```python
from build123d import *

# Parameters (mm, degrees)
BOSS_EXTRUDE1_DEPTH                     = 40
CUT_EXTRUDE3_REACH                      = 349.563
SKETCH2_W                               = 10
SKETCH2_H                               = 8
FILLET1_RADIUS                          = 15
FILLET1_LENGTH                          = 15
SKETCH3_R                               = 5
CUT_EXTRUDE4_DEPTH                      = 15
CUT_EXTRUDE5_REACH                      = 349.394
CBORE_FOR_M5_HEX_HEAD_BOLT1_D           = 10
CBORE_FOR_M5_HEX_HEAD_BOLT1_CBORE_D     = 15
CBORE_FOR_M5_HEX_HEAD_BOLT1_CBORE_DEPTH = 8
CUT_EXTRUDE6_DEPTH                      = 40


with BuildPart() as part:
    # Sketch1 → Boss-Extrude1 (new, symmetric)
    with BuildSketch(Plane.YZ):
        with BuildLine():
            Line((0, 0), (47.251760651, 0))
            ThreePointArc((47.251760651, 0), (58.870710689, 4.252272915), (65, 15))
            Line((65, 15), (196.846599289, 15))
            ThreePointArc((196.846599289, 15), (222.463976204, 19.510639101), (245, 32.5))
            Line((245, 32.5), (280, 32.5))
            Line((280, 32.5), (300, 12.5))
            Line((300, 12.5), (300, -12.5))
            Line((300, -12.5), (340, -12.5))
            Line((340, -12.5), (340, -27.5))
            Line((340, -27.5), (245, -27.5))
            add(Edge.make_bspline(
                [(179, -15), (212.333333333, -15), (211.666666667, -27.5), (245, -27.5)],
                knots=[0, 0, 0, 0, 1, 1, 1, 1], degree=3))
            Line((179, -15), (0, -15))
            Line((0, -15), (0, 0))
        make_face()
    extrude(amount=BOSS_EXTRUDE1_DEPTH, both=True)

    # Cut-Extrude3: up to this face of the body (flat: up to its plane)
    cut_extrude3_end = Plane(part.part.faces().sort_by_distance((0, 292.5, -27.5))[0])
    # Sketch2 → Cut-Extrude3 (cut, up to the picked face)
    with BuildSketch(Plane.XY.offset(32.5), mode=Mode.PRIVATE) as cut_extrude3_sk1:
        with BuildLine():
            Line((15, 202.853988128), (15, 0))
            Line((15, 0), (40, 0))
            Line((40, 0), (40, 47.251760651))
            Line((40, 47.251760651), (40, 245))
            Line((40, 245), (22.765371804, 245))
            Line((22.765371804, 245), (18.407417371, 228.735892638))
            ThreePointArc((18.407417371, 228.735892638), (15.855513863, 215.90660735), (15, 202.853988128))
        make_face()
    cut_extrude3_tool1 = split(extrude(cut_extrude3_sk1.sketch, amount=-CUT_EXTRUDE3_REACH, mode=Mode.PRIVATE), bisect_by=cut_extrude3_end, keep=Keep.BOTH, mode=Mode.PRIVATE)
    # Sketch2 → Cut-Extrude3 (cut, up to the picked face)
    with BuildSketch(Plane.XY.offset(32.5), mode=Mode.PRIVATE) as cut_extrude3_sk2:
        with BuildLine():
            Line((-40, 0), (-15, 0))
            Line((-15, 0), (-15, 202.853988128))
            ThreePointArc((-15, 202.853988128), (-15.855513863, 215.90660735), (-18.407417371, 228.735892638))
            Line((-18.407417371, 228.735892638), (-22.765371804, 245))
            Line((-22.765371804, 245), (-40, 245))
            Line((-40, 245), (-40, 0))
        make_face()
    cut_extrude3_tool2 = split(extrude(cut_extrude3_sk2.sketch, amount=-CUT_EXTRUDE3_REACH, mode=Mode.PRIVATE), bisect_by=cut_extrude3_end, keep=Keep.BOTH, mode=Mode.PRIVATE)
    # Sketch2 → Cut-Extrude3 (cut, up to the picked face)
    with BuildSketch(Plane.XY.offset(32.5), mode=Mode.PRIVATE) as cut_extrude3_sk3:
        Polygon((30, 272), (22.765371804, 245), (40, 245), (40, 272), align=None)
    cut_extrude3_tool3 = split(extrude(cut_extrude3_sk3.sketch, amount=-CUT_EXTRUDE3_REACH, mode=Mode.PRIVATE), bisect_by=cut_extrude3_end, keep=Keep.BOTH, mode=Mode.PRIVATE)
    # Sketch2 → Cut-Extrude3 (cut, up to the picked face)
    with BuildSketch(Plane.XY.offset(32.5), mode=Mode.PRIVATE) as cut_extrude3_sk4:
        Polygon((-40, 272), (-40, 245), (-22.765371804, 245), (-30, 272), align=None)
    cut_extrude3_tool4 = split(extrude(cut_extrude3_sk4.sketch, amount=-CUT_EXTRUDE3_REACH, mode=Mode.PRIVATE), bisect_by=cut_extrude3_end, keep=Keep.BOTH, mode=Mode.PRIVATE)
    # Sketch2 → Cut-Extrude3 (cut, up to the picked face)
    with BuildSketch(Plane.XY.offset(32.5), mode=Mode.PRIVATE) as cut_extrude3_sk5:
        with BuildLine():
            Line((30, 300), (30, 280))
            Line((30, 280), (40, 280))
            Line((40, 280), (40, 340))
            Line((40, 340), (18.5, 340))
            ThreePointArc((18.5, 340), (35.838126061, 329.969422485), (35.78511038, 309.938938469))
            Line((35.78511038, 309.938938469), (35.773706219, 309.919345885))
            Line((35.773706219, 309.919345885), (30, 300))
        make_face()
    cut_extrude3_tool5 = split(extrude(cut_extrude3_sk5.sketch, amount=-CUT_EXTRUDE3_REACH, mode=Mode.PRIVATE), bisect_by=cut_extrude3_end, keep=Keep.BOTH, mode=Mode.PRIVATE)
    # Sketch2 → Cut-Extrude3 (cut, up to the picked face)
    with BuildSketch(Plane.XY.offset(32.5), mode=Mode.PRIVATE) as cut_extrude3_sk6:
        with Locations((35, 276)):
            Rectangle(SKETCH2_W, SKETCH2_H)
    cut_extrude3_tool6 = split(extrude(cut_extrude3_sk6.sketch, amount=-CUT_EXTRUDE3_REACH, mode=Mode.PRIVATE), bisect_by=cut_extrude3_end, keep=Keep.BOTH, mode=Mode.PRIVATE)
    # Sketch2 → Cut-Extrude3 (cut, up to the picked face)
    with BuildSketch(Plane.XY.offset(32.5), mode=Mode.PRIVATE) as cut_extrude3_sk7:
        with Locations((-35, 276)):
            Rectangle(SKETCH2_W, SKETCH2_H)
    cut_extrude3_tool7 = split(extrude(cut_extrude3_sk7.sketch, amount=-CUT_EXTRUDE3_REACH, mode=Mode.PRIVATE), bisect_by=cut_extrude3_end, keep=Keep.BOTH, mode=Mode.PRIVATE)
    # Sketch2 → Cut-Extrude3 (cut, up to the picked face)
    with BuildSketch(Plane.XY.offset(32.5), mode=Mode.PRIVATE) as cut_extrude3_sk8:
        with BuildLine():
            Line((-40, 340), (-40, 280))
            Line((-40, 280), (-30, 280))
            Line((-30, 280), (-30, 300))
            Line((-30, 300), (-35.773706219, 309.919345885))
            Line((-35.773706219, 309.919345885), (-35.78511038, 309.938938469))
            ThreePointArc((-35.78511038, 309.938938469), (-35.838126061, 329.969422485), (-18.5, 340))
            Line((-18.5, 340), (-40, 340))
        make_face()
    cut_extrude3_tool8 = split(extrude(cut_extrude3_sk8.sketch, amount=-CUT_EXTRUDE3_REACH, mode=Mode.PRIVATE), bisect_by=cut_extrude3_end, keep=Keep.BOTH, mode=Mode.PRIVATE)
    add(cut_extrude3_tool1.solids().sort_by(Axis((27.70054, 120.268436, 32.5), (0, 0, -1)))[0], mode=Mode.SUBTRACT)
    add(cut_extrude3_tool2.solids().sort_by(Axis((-27.70054, 120.268436, 32.5), (0, 0, -1)))[0], mode=Mode.SUBTRACT)
    add(cut_extrude3_tool3.solids().sort_by(Axis((33.031192, 257.304616, 32.5), (0, 0, -1)))[0], mode=Mode.SUBTRACT)
    add(cut_extrude3_tool4.solids().sort_by(Axis((-33.031192, 257.304616, 32.5), (0, 0, -1)))[0], mode=Mode.SUBTRACT)
    add(cut_extrude3_tool5.solids().sort_by(Axis((35.537859, 306.308968, 32.5), (0, 0, -1)))[0], mode=Mode.SUBTRACT)
    add(cut_extrude3_tool6.solids().sort_by(Axis((35, 276, 32.5), (0, 0, -1)))[0], mode=Mode.SUBTRACT)
    add(cut_extrude3_tool7.solids().sort_by(Axis((-35, 276, 32.5), (0, 0, -1)))[0], mode=Mode.SUBTRACT)
    add(cut_extrude3_tool8.solids().sort_by(Axis((-35.537859, 306.308968, 32.5), (0, 0, -1)))[0], mode=Mode.SUBTRACT)

    # Fillet1: full round fillet: the end face becomes a half cylinder, R = half its width
    fillet1_face = Plane((0, 0, -7.5), x_dir=(0, 0, -1), z_dir=(0, -1, 0))  # on the end face: x along it, z out of the body
    fillet1_slab = fillet1_face.offset(-FILLET1_RADIUS / 2) * Box(FILLET1_LENGTH, 2 * FILLET1_RADIUS, FILLET1_RADIUS, mode=Mode.PRIVATE)  # the body's end, R deep
    fillet1_round = Plane((0, 15, -7.5), x_dir=(0, -1, 0), z_dir=(0, 0, -1)) * Cylinder(FILLET1_RADIUS, FILLET1_LENGTH, mode=Mode.PRIVATE)  # its axis R under the face
    add(fillet1_slab - fillet1_round, mode=Mode.SUBTRACT)

    # Sketch3 → Cut-Extrude4 (cut)
    with BuildSketch(Plane.XY):
        with Locations((0, 15)):
            Circle(SKETCH3_R)
    extrude(amount=-CUT_EXTRUDE4_DEPTH, mode=Mode.SUBTRACT)

    # Cut-Extrude5: up to this face of the body (flat: up to its plane)
    cut_extrude5_end = Plane(part.part.faces().sort_by_distance((0, 319.72582268, -12.5))[0])
    # Sketch4 → Cut-Extrude5 (cut, up to the picked face)
    with BuildSketch(Plane.XY.offset(32.5), mode=Mode.PRIVATE) as cut_extrude5_sk1:
        with BuildLine():
            Line((-20, 300), (-20, 270))
            ThreePointArc((-20, 270), (-15.606601718, 259.393398282), (-5, 255))
            Line((-5, 255), (5, 255))
            ThreePointArc((5, 255), (15.606601718, 259.393398282), (20, 270))
            Line((20, 270), (20, 300))
            Line((20, 300), (-20, 300))
        make_face()
    cut_extrude5_tool1 = split(extrude(cut_extrude5_sk1.sketch, amount=-CUT_EXTRUDE5_REACH, mode=Mode.PRIVATE), bisect_by=cut_extrude5_end, keep=Keep.BOTH, mode=Mode.PRIVATE)
    add(cut_extrude5_tool1.solids().sort_by(Axis((0, 278.585623, 32.5), (0, 0, -1)))[0], mode=Mode.SUBTRACT)

    # CBORE for M5 Hex Head Bolt1 (through all)
    with Locations(Plane.XY.offset(-12.5)):
        with Locations((-18.46, 320), (18.46, 320), (0, 280)):
            CounterBoreHole(CBORE_FOR_M5_HEX_HEAD_BOLT1_D / 2, CBORE_FOR_M5_HEX_HEAD_BOLT1_CBORE_D / 2, CBORE_FOR_M5_HEX_HEAD_BOLT1_CBORE_DEPTH)

    # Sketch8 → Cut-Extrude6 (cut, symmetric)
    with BuildSketch(Plane.YZ.offset(15)):
        Polygon((63, -7.5), (93, -7.5), (78, 7.5), align=None)
        Polygon((89, 7.5), (119, 7.5), (104, -7.5), align=None)
        Polygon((115, -7.5), (145, -7.5), (130, 7.5), align=None)
        Polygon((156, -7.5), (141, 7.5), (171, 7.5), align=None)
        Polygon((167, -7.5), (197, -7.5), (182, 7.5), align=None)
        Polygon((208, -7.5), (193, 7.5), (223, 7.5), align=None)
    extrude(amount=CUT_EXTRUDE6_DEPTH, both=True, mode=Mode.SUBTRACT)


solid = part.part
```
The model under review builds one solid part; all positions refer to its coordinate system, in mm. A direction names the side the tool comes from. Round coordinates to 2 decimals unless told otherwise and drop trailing zeros. Loops run counter-clockwise (first coordinate to the right, second up) from the corner with the lowest first, then second, coordinate; pieces in that order, holes last. Notation, with made-up numbers: (21, -20) - (73, -20) arc R16 cw to (73, -6) - close; hole circle Ø11 at (22.25, 49). An arc over 180 degrees is marked (long way). Write each question's results on one line, items separated by ' | '. Start each with the question number.
Q1. Take a section at C-C on y = 58. Give the boundary of the cut face in (x, z).
Q2. Take a section at B-B on z = 19. Give the boundary of the cut face in (x, y), plus the area to 3 significant figures.
Q3. Wall thickness on line 1 along X through (y, z) = (320, -17); line 2 along X through (y, z) = (320, -25.25); line 3 along Y through (x, z) = (0, -14): over which ranges is each line inside the solid? List them lowest first. Write a range as [from, to].
Q4. Tool access review of faces 1 (the flat face through (-30, 286, 3)), 2 (the flat face through (0, 91, -15)), 3 (the flat face through (0, 130, -7.5)), 4 (the cylindrical face through (-15.72, 259.51, 10.32)), 5 (the flat face through (-17, 315, -20.5)): name each direction out of +Z, -Z, +X, -X, +Y, -Y from which nothing blocks a thin tool from reaching the whole face with its end or side.
Q5. Insertion check: P1, Ø5, axis at x = -6, z = -4.5, coming from the -Y side; P2, Ø9, axis at x = 5, y = 128.5, coming from the +Z side; P3, Ø4, axis at x = -18.5, z = 25.5, coming from the +Y side; P4, Ø6, axis at x = 0, y = 280, coming from the -Z side. Each pin has a flat end and moves straight along its axis. Give the tip position at first contact, or say it passes through.
Q6. Draft analysis for pull direction Z (two halves, no side actions). For faces 6 (the flat face through (-0.2, 122.6, 0.1)), 7 (the flat face through (0, 130, 15)), 8 (the flat face through (25, 300, 0)), state which applies: pulls with the +Z half, pulls with the -Z half, needs draft (parallel to the pull), parting line crosses it, or undercut.
Q7. Take a section at A-A on y = 135. Give the boundary of the cut face in (x, z).
Data:
1) outline: (-15, -15) - (15, -15) - (15, 3.56) - (-15, 3.56) - close
2) outline: (-30, 272) - (-18.41, 228.74) arc R100 cw to (-16.66, 221.01) - (16.66, 221.01) arc R100 cw to (18.41, 228.74) - (30, 272) - (30, 293.5) - (20, 293.5) - (20, 270) arc R15 cw to (5, 255) - (-5, 255) arc R15 cw to (-20, 270) - (-20, 293.5) - (-30, 293.5) - close | area: 2,210 mm²
3) line 1: x = [-38.5, -25.96], [-10.96, 10.96], [25.96, 38.5] | line 2: x = [-38.5, -23.46], [-13.46, 13.46], [23.46, 38.5] | line 3: y = [0, 10], [20, 272.5], [287.5, 340]
4) face 1: +Z, -Z, -X, -Y | face 2: -Z, +X, -X, -Y | face 3: +X, -X | face 4: +Z, +Y | face 5: +Z
5) P1: stops at y = 0.41 | P2: stops at z = 15 | P3: stops at y = 288.32 | P4: passes through
6) face 6: undercut | face 7: pulls with the +Z half | face 8: needs draft
7) outline: (-15, -15) - (15, -15) - (15, -7.5) - (-15, -7.5) - close; (-15, 2.5) - (15, 2.5) - (15, 15) - (-15, 15) - close
